Geometry: final body of the model. Coordinates: model frame, mm. Coordinates: 2 decimals unless noted, no trailing zeros. Write each loop counter-clockwise with the first axis right and the second up, starting at its lowest first coordinate (ties: lowest second). Pieces come first, ordered by that corner, then holes.
from build123d import *

# Parameters (mm, degrees)
ESBO_O1_W                = 200
ESBO_O1_H                = 50
RESSALTO_EXTRUS_O1_DEPTH = 10
FILETE1_R                = 5
FUROS_GUIA_COM_20_0MM1_D = 20


with BuildPart() as part:
    # Esboço1 → Ressalto-extrusão1 (new body)
    with BuildSketch(Plane.XY):
        with Locations((100, 25)):
            Rectangle(ESBO_O1_W, ESBO_O1_H)
    extrude(amount=RESSALTO_EXTRUS_O1_DEPTH)

    # Filete1
    filete1_edges = [part.edges().sort_by_distance(p)[0] for p in [
        (100, 50, 10),
        (0, 25, 10),
        (100, 0, 10),
        (0, 25, 0),
        (100, 50, 0),
        (200, 25, 0),
        (100, 0, 0),
        (0, 0, 5),
        (0, 50, 5),
        (200, 50, 5),
        (200, 0, 5),
        (200, 25, 10),
    ]]
    fillet(filete1_edges, radius=FILETE1_R - 0.0001)  # a hair under: the kernel refuses the full size

    # Furos-guia com Ø20.0mm1 (through all)
    with Locations(Plane.XY.offset(10)):
        with Locations((45, 25.206865572), (155, 25.206865572)):
            Hole(FUROS_GUIA_COM_20_0MM1_D / 2)


solid = part.part
Item 1: Pull-direction query (Y, two-part tool) for faces 1 (the cylindrical face through (54.99, 25.65, 4.93)), 2 (the cylindrical face through (1, 25, 8)), 3 (the cylindrical face through (101, 49, 2)); classes: released by +Y, released by -Y, zero draft, split by the parting line, or undercut.
Derived:
face 1: undercut
face 2: zero draft
face 3: released by +Y
Item 2: Section B-B, the plane y = 28.5. State how many separate pieces and enclosed holes the cut face has, plus the area to 3 significant figures.
Derived:
separate pieces: 3
enclosed holes: 0
area: 1,600 mm2
Item 3: Material intervals for probe 1 along X at (y, z) = (25, 5.5); probe 2 along Y at (x, z) = (45, 5.5); probe 3 along X at (y, z) = (34, 4.25), sorted ascending.
Derived:
probe 1: x = 0.03 to 35, 55 to 145, 165 to 199.97
probe 2: y = 0.03 to 15.21, 35.21 to 49.97
probe 3: x = 0.06 to 40.24, 49.76 to 150.24, 159.76 to 199.94
Item 4: Pin query (flat end, axial travel): pin 1 (6 mm diameter, centred on y = 30, z = 9, fed in from -X); pin 2 (1.5 mm diameter, centred on x = 179.5, z = 8, fed in from +Y). Return the tip coordinate at first contact, or that it passes through.
Derived:
pin 1: stops at x = 0.1
pin 2: stops at y = 49.47
Item 5: Section C-C, the plane z = 2. Output: boundary loops of the cut face in (x, y).
Derived:
outline: (1, 5) arc R4 ccw to (5, 1) - (195, 1) arc R4 ccw to (199, 5) - (199, 45) arc R4 ccw to (195, 49) - (5, 49) arc R4 ccw to (1, 45) - close; hole circle Ø20 at (45, 25.21); hole circle Ø20 at (155, 25.21)
